Design review of the part shown in the three views and the two pictorial views. Dimensions are in mm from the part's minimum x, y and z. Coordinates: 2 decimals unless noted, no trailing zeros. Loops run counter-clockwise (first coordinate to the right, second up) from the corner with the lowest first, then second, coordinate; pieces in that order, holes last. Notation, with made-up numbers: (89, 51.25) - (101, 51.25) arc R11 cw to (101, 70.25) - close; hole circle Ø3 at (57.5, 82.25). An arc over 180 degrees is marked (long way). One line per question, with ' | ' between items.
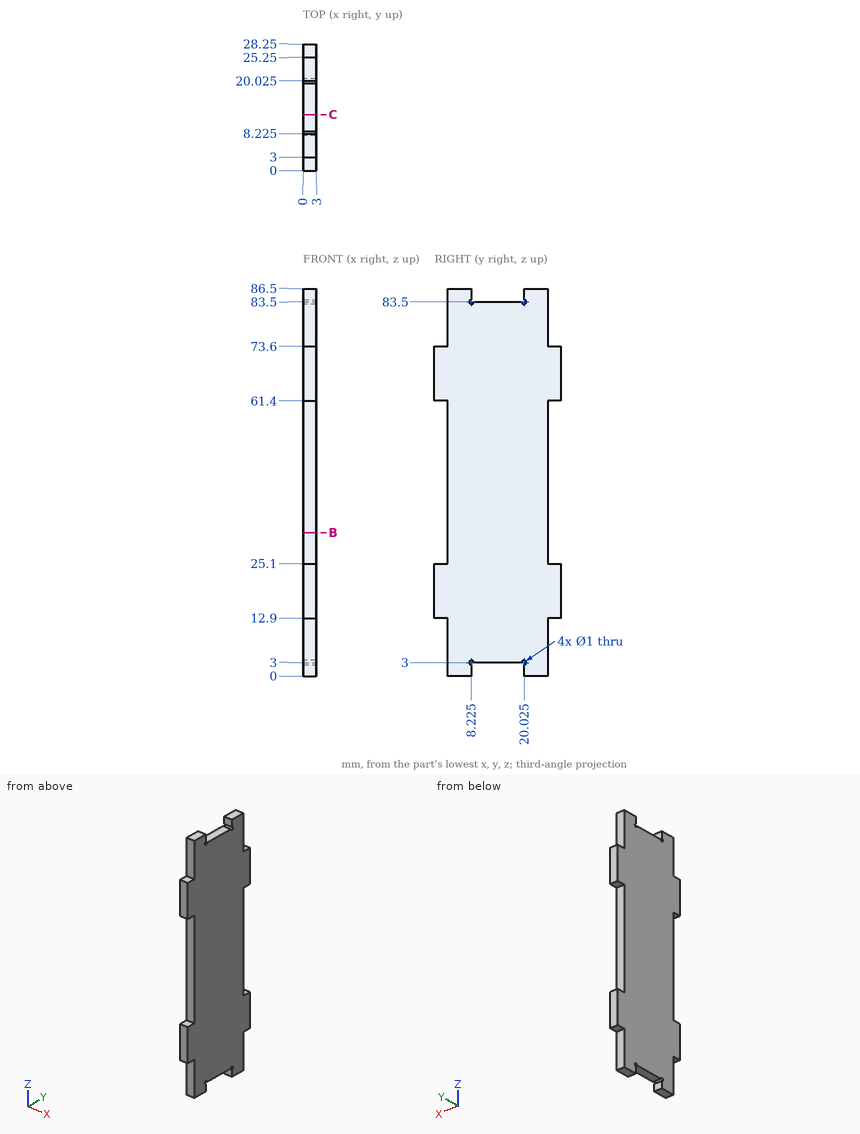
Q1. To check wall thickness, follow line 1 along Z through (x, y) = (0.4, 2); line 2 along Z through (x, y) = (1.05, 20.25); line 3 along Y through (x, z) = (2.35, 46). State the ranges of each line that lie inside material, in increasing order.
Returned:
line 1: z = 12.9 to 25.1, 61.4 to 73.6 | line 2: z = 0 to 2.55, 3.45 to 83.05, 83.95 to 86.5 | line 3: y = 3 to 25.25
Q2. Take a section at C-C (y = 12.5). Give the boundary of the cut face in (x, z).
Returned:
outline: (0, 3) - (3, 3) - (3, 83.5) - (0, 83.5) - close
Q3. For pin 1 (1.5 mm diameter, centred on x = 1, z = 34.5, fed in from +Y); pin 2 (0.9 mm diameter, centred on y = 20.025, z = 83.5, fed in from +X); pin 3 (1.5 mm diameter, centred on x = 1.5, y = 27, fed in from -Z); pin 4 (0.9 mm diameter, centred on x = 2, y = 2, fed in from +Z), all flat-tipped, find the tip position at first contact; note any pin that passes through.
Returned:
pin 1: stops at y = 25.25 | pin 2: passes through | pin 3: stops at z = 12.9 | pin 4: stops at z = 73.6
Q4. Take a section at B-B (z = 32). Give the boundary of the cut face in (x, y).
Returned:
outline: (0, 3) - (3, 3) - (3, 25.25) - (0, 25.25) - close
